```python
from build123d import *

# Parameters (mm, degrees)
F0_R     = 2.9972
F1_DEPTH = 76.962
F1_TAPER = 1
F4_R     = 1.27
F5_DEPTH = 3.81


with BuildPart() as f1:
    # F0 (on Front) → F1 (new body)
    with BuildSketch(Plane.XZ):
        Circle(F0_R)
    extrude(amount=F1_DEPTH, taper=F1_TAPER)

    # F2 (on Right) → F3 (revolve)
    with BuildSketch(Plane.YZ):
        with BuildLine():
            Line((0.2946257891, 0.4991786979), (0, 0))
            Line((0, 0), (-1.5448811736, -2.6174618826))
            Line((-1.5448811736, -2.6174618826), (0, -3.529283314))
            ThreePointArc((0, -3.529283314), (1.1892758064, -3.4725018248), (2.0940375895, -2.6985462724))
            Line((2.0940375895, -2.6985462724), (6.6074357329, 4.9484157097))
            Line((6.6074357329, 4.9484157097), (3.8731704317, 6.5622367229))
            Line((3.8731704317, 6.5622367229), (0.2946257891, 0.4991786979))
        make_face()
    revolve(axis=Axis((0, 1.9365852158, 3.2811183614), (0, 0.5082900829, 0.8611859216)))

    # F4 (on face) → F5 (join)
    with BuildSketch(Plane.XZ.offset(76.962)):
        Circle(F4_R)
    extrude(amount=F5_DEPTH)


solid = f1.part
```
Work out the finished part from the listing and answer in its coordinate system (mm). A direction names the side the tool comes from. Give positions to 0.01 mm unless a question says otherwise; leave off trailing zeros. Loops run counter-clockwise (first coordinate to the right, second up) from the corner with the lowest first, then second, coordinate; pieces in that order, holes last. Notation, with made-up numbers: (81.5, -1) -> (139.5, -1) arc R16 cw to (139.5, 8) -> close; hole circle Ø10 at (62, 57). An arc over 180 degrees is marked (long way). One line per question, with ' | ' between items. Start each with the question number.
1) Each of these flat-tipped pins is pushed along its axis until it touches: pin 1 (3 mm diameter, centred on y = -59, z = 5, fed in from -X); pin 2 (1 mm diameter, centred on x = -2, y = -52.5, fed in from -Z); pin 3 (1 mm diameter, centred on y = -12, z = -2.5, fed in from -X); pin 4 (1 mm diameter, centred on x = 0, y = -58, fed in from -Z). Where does it stop, or does it pass through?
2) For faces 1 (the face through (-0.954, 4.256, 1.253)), 2 (the face through (-0.03, -0.73, -3.1)), 3 (the face through (-0.17, -78.84, 1.26)), determine the directions among +Z, -Z, +X, -X, +Y, -Y from which every point of the face is accessible in a straight line to the end or side of a thin tool.
3) Section B-B, the plane y = -63 is taken. Determine the outline of the cut face in (x, z), then the cut area to 3 significant figures.
4) Section A-A, the plane y = -72 is taken. Determine the outline of the cut face in (x, z).
5) Straight lines are drawn through the part: L1, parallel to X at y = 2, z = 4; L2, parallel to X at y = -2, z = 1; L3, parallel to Z at x = 0.5, y = -53. For each, find the intervals that lie inside material, in ascending order.
Resolved:
1) pin 1: through | pin 2: z = -1.44 | pin 3: x = -1.94 | pin 4: z = -1.99
2) face 1: none | face 2: -Z, -Y | face 3: -Y
3) outline: circle Ø3.8 at (0, 0) | area: 11.3 mm2
4) outline: circle Ø3.48 at (0, 0)
5) L1: -3.16 to 3.16 | L2: -2.79 to 2.79 | L3: -2.01 to 2.01
